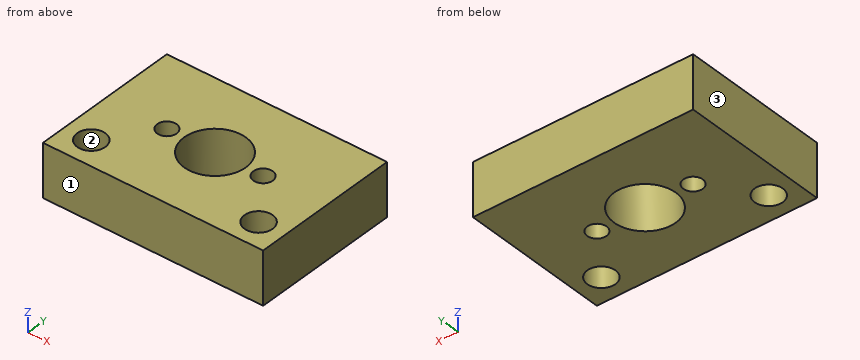
```python
from build123d import *

# Parameters (mm, degrees)
SKIZZE1_W                        = 25
SKIZZE1_H                        = 17
AUFSATZ_LINEAR_AUSTRAGEN1_DEPTH  = 6
F_3_2_3_2_DURCHMESSER_BOHRUNG1_D = 3.2
F_7_0_7_DURCHMESSER_BOHRUNG1_D   = 7
F_2_2_2_2_DURCHMESSER_BOHRUNG1_D = 2.2


with BuildPart() as part:
    # Skizze1 → Aufsatz-Linear austragen1 (new body)
    with BuildSketch(Plane.XY):
        Rectangle(SKIZZE1_W, SKIZZE1_H)
    extrude(amount=AUFSATZ_LINEAR_AUSTRAGEN1_DEPTH)

    # Ø3.2 (3.2) Durchmesser Bohrung1 (through all)
    with Locations(Plane.XY.offset(6)):
        with Locations((-9.5, -5.5), (9.5, -5.5)):
            Hole(F_3_2_3_2_DURCHMESSER_BOHRUNG1_D / 2)

    # Ø7.0 (7) Durchmesser Bohrung1 (through all)
    with Locations(Plane.XY.offset(6)):
        with Locations((0, 0)):
            Hole(F_7_0_7_DURCHMESSER_BOHRUNG1_D / 2)

    # Ø2.2 (2.2) Durchmesser Bohrung1 (through all)
    with Locations(Plane.XY.offset(6)):
        with Locations((-5.46, 0), (5.46, 0)):
            Hole(F_2_2_2_2_DURCHMESSER_BOHRUNG1_D / 2)


solid = part.part
```
Could you check a few things on this model? Use its own coordinates, in mm. Face numbers are marked on the shaded views. Coordinates: 2 decimals unless noted, no trailing zeros. Order: outer loops, then holes, each group sorted by start corner. A loop starts at its lowest first (then second) coordinate and runs counter-clockwise, first axis right, second up. Notation, with made-up numbers: M -32,25.25 L 2,25.25 A35 cw 2,63.25 Z; hole C 32,14 d11. An arc over 180 degrees is marked long. Use one line per item in the form item = value. Start each with the question number.
1. For pin 1 (3 mm diameter, centred on x = -9.5, y = -5.5, fed in from -Z), with a flat end and sliding along its axis, tell me the tip position at first contact or that it passes through.
2. Suppose I cut it at C-C on z = 4.8. Write out the boundary of the cut face in (x, y), then the cut area to 3 significant figures.
3. Suppose I cut it at B-B on x = 0. Write out the boundary of the cut face in (y, z).
4. Suppose I cut it at A-A on y = 0. Write out the boundary of the cut face in (x, z).
5. Please list where these lines run through material, in increasing order: line 1 (Y direction, x = -9.5, z = 2); line 2 (X direction, y = 1, z = 1.15); line 3 (X direction, y = -2.5, z = 5.75).
6. We'd pull the mould along X, two halves only. Please class the marked faces 1, 2 and 3: +X half, -X half, draft (parallel to the pull), parting line (faces both ways), or undercut.
7. Suppose I cut it at D-D on y = -5.5. Write out the boundary of the cut face in (x, z).
Geometry says:
q1.pin_1 = through
q2.outline = M -12.5,-8.5 L 12.5,-8.5 L 12.5,8.5 L -12.5,8.5 Z; hole C -9.5,-5.5 d3.2; hole C -5.46,0 d2.2; hole C 0,0 d7; hole C 5.46,0 d2.2; hole C 9.5,-5.5 d3.2
q2.area = 363 mm^2
q3.outline = M -8.5,0 L -3.5,0 L -3.5,6 L -8.5,6 Z; M 3.5,0 L 8.5,0 L 8.5,6 L 3.5,6 Z
q4.outline = M -12.5,0 L -6.56,0 L -6.56,6 L -12.5,6 Z; M -4.36,0 L -3.5,0 L -3.5,6 L -4.36,6 Z; M 3.5,0 L 4.36,0 L 4.36,6 L 3.5,6 Z; M 6.56,0 L 12.5,0 L 12.5,6 L 6.56,6 Z
q5.line_1 = -8.5 to -7.1, -3.9 to 8.5
q5.line_2 = -12.5 to -5.92, -5 to -3.35, 3.35 to 5, 5.92 to 12.5
q5.line_3 = -12.5 to -2.45, 2.45 to 12.5
q6.face_1 = draft
q6.face_2 = undercut
q6.face_3 = -X half
q7.outline = M -12.5,0 L -11.1,0 L -11.1,6 L -12.5,6 Z; M -7.9,0 L 7.9,0 L 7.9,6 L -7.9,6 Z; M 11.1,0 L 12.5,0 L 12.5,6 L 11.1,6 Z
